Verification items for this drawing (mm, ordinates from the low corner). A direction names the side the tool comes from. Give positions to 0.01 mm unless a question says otherwise; leave off trailing zeros. Loops run counter-clockwise (first coordinate to the right, second up) from the corner with the lowest first, then second, coordinate; pieces in that order, holes last. Notation, with made-up numbers: (52.25, 30) -> (88.25, 30) arc R14 cw to (88.25, 35) -> close; hole circle Ø5 at (76, -29). An arc over 180 degrees is marked (long way). Write each question's results on one line, items separated by ' | '. Start each with the question number.
1) Scan lines: line 1 (Y direction, x = 2.25, z = 4); line 2 (Z direction, x = 5.75, y = 6); line 3 (X direction, y = 9.5, z = 17). Record each from-to range of solid material in increasing order. Write a range as from..to.
2) Set-up check for the marked faces 1, 2 and 3: record each of +Z, -Z, +X, -X, +Y, -Y from which the full face is reachable in a straight line by a thin tool's end or side.
3) Sectioned sample at C-C on y = 14.5. Record the cut outline in (x, z) (1 decimal), then the cut area to 3 significant figures.
4) Depth check by flat-ended pin: pin 1 (3 mm diameter, centred on y = 15.5, z = 13.5, fed in from -X); pin 2 (9 mm diameter, centred on x = 9.5, y = 3.5, fed in from +Z); pin 3 (10 mm diameter, centred on y = 4, z = 13, fed in from +X). Enter the tip coordinate at first touch or a pass-through.
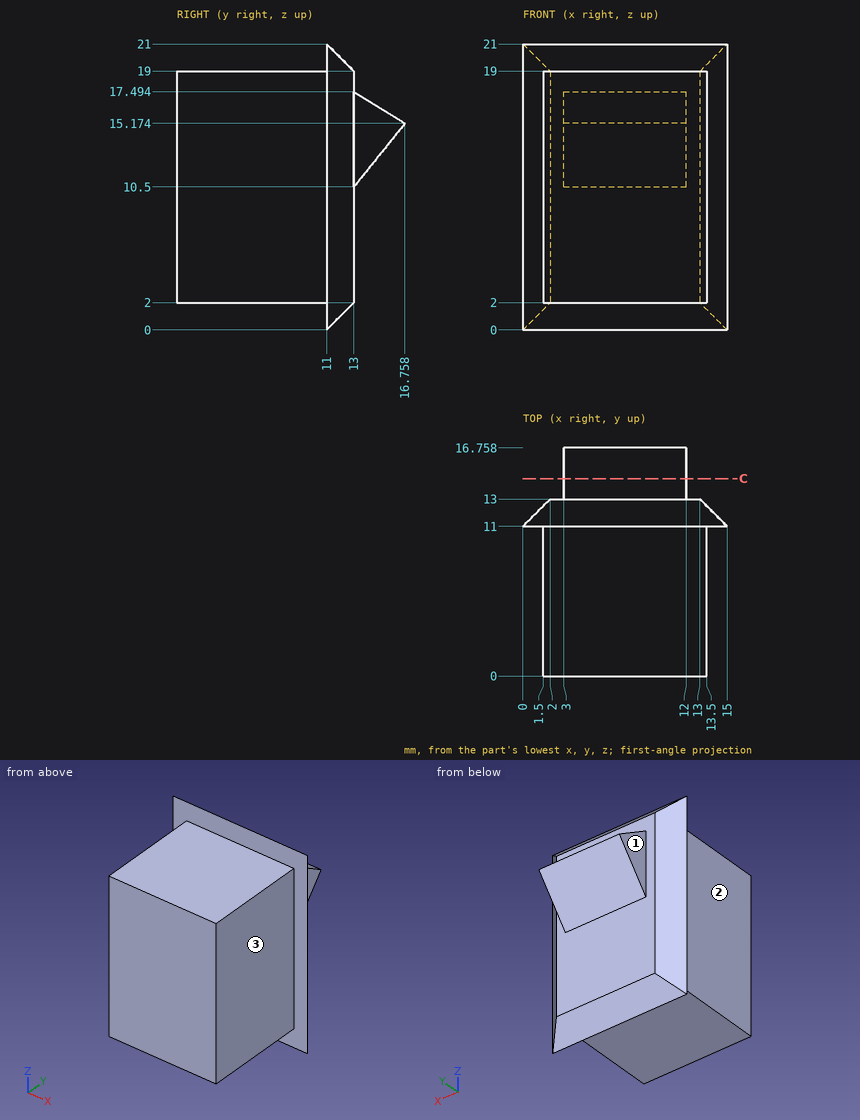
Result:
1) line 1: 0..13 | line 2: 2..19 | line 3: 1.5..13.5
2) face 1: +Z, -Z, -X, +Y | face 2: +Z, -Z, -X, -Y | face 3: +Z, -Z, +X, -Y
3) outline: (3, 12.4) -> (12, 12.4) -> (12, 16.6) -> (3, 16.6) -> close | area: 37.8 mm^2
4) pin 1: x = 3 | pin 2: z = 19 | pin 3: x = 13.5
